```python
from build123d import *

# Parameters (mm, degrees)
SKETCH1_W                    = 41.275
SKETCH1_H                    = 2.58826
BASE_FLANGE1_DEPTH           = 82.55
EDGE_FLANGE1_STRIP_W         = 16.70304
EDGE_FLANGE1_STRIP_H         = 2.58826
EDGE_FLANGE1_STRIP_CUT_DEPTH = 41.275
EDGE_FLANGE1_DEPTH           = 41.275
EDGE_FLANGE1_START           = 2.58826
EDGE_FLANGE1_FLAT_DEPTH      = 2.58826
EDGE_FLANGE2_STRIP_W         = 16.70304
EDGE_FLANGE2_STRIP_H         = 2.58826
EDGE_FLANGE2_STRIP_CUT_DEPTH = 41.275
EDGE_FLANGE2_DEPTH           = 41.275
EDGE_FLANGE2_START           = 2.58826
EDGE_FLANGE2_FLAT_DEPTH      = 2.58826
F_1_4_CLEARANCE_HOLE1_D      = 6.7564
F_10_0_1935_DIAMETER_HOLE1_D = 4.9149
SKETCH19_W                   = 9.191105822
SKETCH19_H                   = 31.75
CUT_EXTRUDE1_DEPTH           = 416.675275559
FILLET2_START                = -2.58826
FILLET2_DEPTH                = 87.72652
FILLET2_2_DEPTH              = 2.58826
FILLET2_START_2              = 82.55
FILLET2_3_DEPTH              = 2.58826


with BuildPart() as part:
    # Base-Flange1: sheet metal written as solids
    # Sketch1 → Base-Flange1 (new body)
    with BuildSketch(Plane(origin=(0, 0, 0), x_dir=(0, 0, -1), z_dir=(1, 0, 0))):
        with Locations((-330.343394178, 62.20587)):
            Rectangle(SKETCH1_W, SKETCH1_H)
    extrude(amount=BASE_FLANGE1_DEPTH)

    # Edge-Flange1: sheet metal written as solids
    # Edge-Flange1 strip (on a plane across the edge) → Edge-Flange1 strip cut (cut)
    with BuildSketch(Plane(origin=(82.55, 60.91174, 309.705894178), x_dir=(-1, 0, 0), z_dir=(0, 0, 1))):
        with Locations((-5.17652, -1.29413)):
            Rectangle(EDGE_FLANGE1_STRIP_W, EDGE_FLANGE1_STRIP_H)
    extrude(amount=EDGE_FLANGE1_STRIP_CUT_DEPTH, mode=Mode.SUBTRACT)

    # Edge-Flange1 bend section (on a plane across the edge) → Edge-Flange1 (add)
    with BuildSketch(Plane(origin=(82.55, 60.91174, 309.705894178), x_dir=(-1, 0, 0), z_dir=(0, 0, 1))):
        with BuildLine():
            Line((-2.58826, 3.175), (0, 3.175))
            ThreePointArc((0, 3.175), (0.92993597, 0.92993597), (3.175, 0))
            Line((3.175, 0), (3.175, -2.58826))
            ThreePointArc((3.175, -2.58826), (-0.900240228, -0.900240228), (-2.58826, 3.175))
        make_face()
    extrude(amount=EDGE_FLANGE1_DEPTH)

    # Edge-Flange1 profile (on flange) → Edge-Flange1 flat (add)
    with BuildSketch(Plane(origin=(82.55, 60.91174, 0), x_dir=(0, 0, 1), z_dir=(1, 0, 0)).offset(EDGE_FLANGE1_START)):
        Polygon((350.980894178, 3.175), (350.980894178, 12.7), (350.980894178, 29.16174), (401.32, 29.16174), (401.32, 60.91174), (309.705894178, 60.91174), (309.705894178, 12.7), (309.705894178, 3.175), align=None)
    extrude(amount=-EDGE_FLANGE1_FLAT_DEPTH)

    # Edge-Flange2: sheet metal written as solids
    # Edge-Flange2 strip (on a plane across the edge) → Edge-Flange2 strip cut (cut)
    with BuildSketch(Plane(origin=(0, 60.91174, 350.980894178), x_dir=(1, 0, 0), z_dir=(0, 0, -1))):
        with Locations((-5.17652, -1.29413)):
            Rectangle(EDGE_FLANGE2_STRIP_W, EDGE_FLANGE2_STRIP_H)
    extrude(amount=EDGE_FLANGE2_STRIP_CUT_DEPTH, mode=Mode.SUBTRACT)

    # Edge-Flange2 bend section (on a plane across the edge) → Edge-Flange2 (add)
    with BuildSketch(Plane(origin=(0, 60.91174, 350.980894178), x_dir=(1, 0, 0), z_dir=(0, 0, -1))):
        with BuildLine():
            Line((-2.58826, 3.175), (0, 3.175))
            ThreePointArc((0, 3.175), (0.92993597, 0.92993597), (3.175, 0))
            Line((3.175, 0), (3.175, -2.58826))
            ThreePointArc((3.175, -2.58826), (-0.900240228, -0.900240228), (-2.58826, 3.175))
        make_face()
    extrude(amount=EDGE_FLANGE2_DEPTH)

    # Edge-Flange2 profile (on flange) → Edge-Flange2 flat (add)
    with BuildSketch(Plane(origin=(0, 60.91174, 0), x_dir=(0, 0, -1), z_dir=(-1, 0, 0)).offset(EDGE_FLANGE2_START)):
        Polygon((-350.980894178, 12.7), (-350.980894178, 3.175), (-309.705894178, 3.175), (-309.705894178, 12.7), (-309.705894178, 60.91174), (-401.32, 60.91174), (-401.32, 29.16174), (-350.980894178, 29.16174), align=None)
    extrude(amount=-EDGE_FLANGE2_FLAT_DEPTH)

    # 1/4 Clearance Hole1 (through all)
    with Locations(Plane.ZY.offset(2.58826)):
        with Locations((382.603894178, 22.225)):
            Hole(F_1_4_CLEARANCE_HOLE1_D / 2)

    # #10 (0.1935) Diameter Hole1 (through all)
    with Locations(Plane(origin=(0, 63.5, 0), x_dir=(1, 0, 0), z_dir=(0, 1, 0))):
        with Locations((15.875, -318.644154178), (15.875, -341.455894178), (66.675, -341.455894178), (66.675, -318.644154178)):
            Hole(F_10_0_1935_DIAMETER_HOLE1_D / 2)

    # Sketch19 → Cut-Extrude1 (cut, through all)
    with BuildSketch(Plane.ZY.offset(2.58826)):
        with Locations((396.724447089, 15.875)):
            Rectangle(SKETCH19_W, SKETCH19_H)
    extrude(amount=-CUT_EXTRUDE1_DEPTH, mode=Mode.SUBTRACT)

    # Fillet2: read off the stored shape, not the designer's step
    # Fillet2 outline → Fillet2 (cut)
    with BuildSketch(Plane.YZ.offset(FILLET2_START)):
        with BuildLine():
            ThreePointArc((0, 365.97937835), (0.084934458, 366.708843873), (0.335193669, 367.399281516))
            Line((0.335193669, 367.399281516), (11.822451583, 390.373797344))
            ThreePointArc((11.822451583, 390.373797344), (12.993061633, 391.654710495), (14.662257914, 392.128894178))
            Line((14.662257914, 392.128894178), (0, 392.128894178))
            Line((0, 392.128894178), (0, 365.97937835))
        make_face()
        with BuildLine():
            ThreePointArc((3.175, 309.705894178), (0.92993597, 310.635830148), (0, 312.880894178))
            Line((0, 312.880894178), (0, 309.705894178))
            Line((0, 309.705894178), (3.175, 309.705894178))
        make_face()
        with BuildLine():
            Line((31.75, 392.128894178), (28.575, 392.128894178))
            ThreePointArc((28.575, 392.128894178), (30.820064031, 391.198958209), (31.75, 388.953894178))
            Line((31.75, 388.953894178), (31.75, 392.128894178))
        make_face()
    extrude(amount=FILLET2_DEPTH, mode=Mode.SUBTRACT)

    # Fillet2 2 outline → Fillet2 2 (add)
    with BuildSketch(Plane.YZ.offset(FILLET2_START)):
        with BuildLine():
            ThreePointArc((34.925, 350.980894178), (32.67993597, 351.910830148), (31.75, 354.155894178))
            Line((31.75, 354.155894178), (31.75, 350.980894178))
            Line((31.75, 350.980894178), (34.925, 350.980894178))
        make_face()
    extrude(amount=FILLET2_2_DEPTH)

    # Fillet2 3 outline → Fillet2 3 (add)
    with BuildSketch(Plane.YZ.offset(FILLET2_START_2)):
        with BuildLine():
            ThreePointArc((34.925, 350.980894178), (32.67993597, 351.910830148), (31.75, 354.155894178))
            Line((31.75, 354.155894178), (31.75, 350.980894178))
            Line((31.75, 350.980894178), (34.925, 350.980894178))
        make_face()
    extrude(amount=FILLET2_3_DEPTH)


solid = part.part
```
Check sheet for the modelled part. Datum: model origin and axes. Units: mm. A direction names the side the tool comes from. Coordinates: 2 decimals unless noted, no trailing zeros. Loops run counter-clockwise (first coordinate to the right, second up) from the corner with the lowest first, then second, coordinate; pieces in that order, holes last.
1) Gauge pin test, flat ends, axial feed: pin 1 (5.5 mm diameter, centred on y = 22.22, z = 382.6, fed in from +X); pin 2 (6.5 mm diameter, centred on x = 66.68, z = 341.46, fed in from +Y); pin 3 (10 mm diameter, centred on x = 45.5, z = 328.5, fed in from -Y); pin 4 (3 mm diameter, centred on x = -1, z = 370, fed in from +Y). Record the tip position at first contact, or that the pin passes through.
2) Release check for a two-part mould opening along Y. For faces 4 (the face through (83.405, 61.857, 330.054)), 5 (the face through (83.86, 22.37, 385.98)), 6 (the face through (81.6, 60, 330.1)) record: released by +Y, released by -Y, zero draft, split by the parting line, or undercut.
3) Sectioned sample at D-D (x = 28). Record the boundary of the cut face in (y, z), and give its area (3 significant figures).
4) Sectioned sample at C-C (z = 346). Record the boundary of the cut face in (x, y) (3 decimals).
5) Access from +Z, -Z, +X, -X, +Y, -Y to the whole of each face (thin tool, end or side, straight path). Record for faces 1 (the face through (-1, 0, 339)), 2 (the face through (-1, 31.75, 372)), 3 (the face through (0, 22, 342)).
6) Sectioned sample at B-B (z = 375.5). Record the boundary of the cut face in (x, y), and give its area (3 significant figures).
7) Sectioned sample at A-A (y = 39.5). Record the boundary of the cut face in (x, z), and give its area (3 significant figures).
8) Material ranges on probe 1 along Z at (x, y) = (16, 61); probe 2 along X at (y, z) = (51, 325); probe 3 along Y at (x, z) = (6, 330.5), recorded low to high.
Check sheet entries:
1. pin 1: passes through
1. pin 2: stops at y = 63.5
1. pin 3: stops at y = 60.91
1. pin 4: stops at y = 31.75
2. face 4: released by +Y
2. face 5: undercut
2. face 6: released by -Y
3. outline: (60.91, 309.71) - (63.5, 309.71) - (63.5, 350.98) - (60.91, 350.98) - close
3. area: 107 mm2
4. outline: (-2.588, 0) - (0, 0) - (0, 57.737) arc R3.175 cw to (3.175, 60.912) - (79.375, 60.912) arc R3.175 cw to (82.55, 57.737) - (82.55, 0) - (85.138, 0) - (85.138, 57.737) arc R5.763 ccw to (79.375, 63.5) - (3.175, 63.5) arc R5.763 ccw to (-2.588, 57.737) - close
5. face 1: +Z, -Z, +X, -X, -Y
5. face 2: +Z, +X, -X, +Y
5. face 3: +Z, -Z, -Y
6. outline: (-2.59, 4.39) - (0, 4.39) - (0, 31.75) - (-2.59, 31.75) - close; (82.55, 4.39) - (85.14, 4.39) - (85.14, 31.75) - (82.55, 31.75) - close
6. area: 142 mm2
7. outline: (-2.59, 309.71) - (0, 309.71) - (0, 350.98) - (-2.59, 350.98) - close; (82.55, 309.71) - (85.14, 309.71) - (85.14, 350.98) - (82.55, 350.98) - close
7. area: 214 mm2
8. probe 1: z = 309.71 to 316.19, 321.1 to 339, 343.91 to 350.98
8. probe 2: x = -2.59 to 0, 82.55 to 85.14
8. probe 3: y = 60.91 to 63.5
